```python
from build123d import *

# Parameters (mm, degrees)
SKETCH_1_R      = 3.75
SKETCH_1_W      = 18.3
SKETCH_1_H      = 8.8
EXTRUDE_1_DEPTH = 1000


with BuildPart() as part:
    # Эскиз1 → Бобышка-Вытянуть1 (new body)
    with BuildSketch(Plane.XY):
        Polygon((-30, 7.2), (-30, 20), (-7.2, 20), (-4.3, 20), (-4.3, 16.1), (-7.2, 16.1), (-7.2, 8.7), (-4.3, 8.7), (-4.3, 5.7), (4.3, 5.7), (4.3, 8.7), (7.2, 8.7), (7.2, 16.1), (4.3, 16.1), (4.3, 20), (7.2, 20), (30, 20), (30, 7.2), (30, 4.3), (26.1, 4.3), (26.1, 7.2), (18.7, 7.2), (18.7, 4.3), (15.7, 4.3), (15.7, -4.3), (18.7, -4.3), (18.7, -7.2), (26.1, -7.2), (26.1, -4.3), (30, -4.3), (30, -7.2), (30, -20), (7.2, -20), (4.3, -20), (4.3, -16.1), (7.2, -16.1), (7.2, -8.7), (4.3, -8.7), (4.3, -5.7), (-4.3, -5.7), (-4.3, -8.7), (-7.2, -8.7), (-7.2, -16.1), (-4.3, -16.1), (-4.3, -20), (-7.2, -20), (-30, -20), (-30, -7.2), (-30, -4.3), (-26.1, -4.3), (-26.1, -7.2), (-18.7, -7.2), (-18.7, -4.3), (-15.7, -4.3), (-15.7, 4.3), (-18.7, 4.3), (-18.7, 7.2), (-26.1, 7.2), (-26.1, 4.3), (-30, 4.3), align=None)
        Circle(SKETCH_1_R, mode=Mode.SUBTRACT)
        Polygon((-13.2, -7.2), (-13.2, 7.2), (-9, 7.2), (-9, 4.4), (-5.7, 4.4), (-5.7, -4.4), (-9, -4.4), (-9, -7.2), align=None, mode=Mode.SUBTRACT)
        with Locations((-18.85, 13.6)):
            Rectangle(SKETCH_1_W, SKETCH_1_H, mode=Mode.SUBTRACT)
        with Locations((-18.85, -13.6)):
            Rectangle(SKETCH_1_W, SKETCH_1_H, mode=Mode.SUBTRACT)
        with Locations((18.85, -13.6)):
            Rectangle(SKETCH_1_W, SKETCH_1_H, mode=Mode.SUBTRACT)
        Polygon((9, 4.4), (5.7, 4.4), (5.7, -4.4), (9, -4.4), (9, -7.2), (13.2, -7.2), (13.2, 7.2), (9, 7.2), align=None, mode=Mode.SUBTRACT)
        with Locations((18.85, 13.6)):
            Rectangle(SKETCH_1_W, SKETCH_1_H, mode=Mode.SUBTRACT)
    extrude(amount=EXTRUDE_1_DEPTH)


solid = part.part
```
Read the model definition and answer for the solid it produces. Units are mm, in the model's axes. A direction names the side the tool comes from. Give positions to 0.01 mm unless a question says otherwise; leave off trailing zeros. Write item = value, one per line. Start each with the question number.
Item 1: This flat-tipped pin is pushed along its axis until it touches: P1, Ø1, axis at y = -2, z = 208.5, coming from the +X side. Where does it stop, or does it pass through?
Item 2: Find the intervals of material crossed by probe 1 along Y at (x, z) = (-10.5, 774.5); probe 2 along X at (y, z) = (12, 260); probe 3 along Y at (x, z) = (-18, 487), in increasing order. Write a range as [from, to].
Item 3: A tool of negligible diameter and unlimited length cuts with its end or side. For faces 5 (the flat face through (-30, -12, 493)), 6 (the flat face through (19, 18, 493)), from which of +Z, -Z, +X, -X, +Y, -Y can it reach the whole face along a straight path? Write none if from no direction.
Item 4: Find section A-A (z = 170.5). State how many separate pieces and enclosed holes the cut face has, then the cut area to 3 significant figures.
Item 5: The mould has two halves that part along X. Classify faces 1 (the flat face through (19, 9.2, 493)), 2 (the flat face through (17, -20, 493)), 3 (the flat face through (30, -12, 493)), 4 (the flat face through (19, -9.2, 493)): +X half, -X half, draft (parallel to the pull), parting line (faces both ways), or undercut.
Response:
q1.P1 = 15.7
q2.probe_1 = [-20, -18], [-9.2, -7.2], [7.2, 9.2], [18, 20]
q2.probe_2 = [-30, -28], [-9.7, -7.2], [7.2, 9.7], [28, 30]
q2.probe_3 = [-20, -18], [-9.2, -4.3], [4.3, 9.2], [18, 20]
q3.face_5 = +Z, -Z, -X, +Y, -Y
q3.face_6 = +Z, -Z
q4.separate_pieces = 1
q4.enclosed_holes = 7
q4.area = 869 mm²
q5.face_1 = undercut
q5.face_2 = draft
q5.face_3 = +X half
q5.face_4 = undercut
